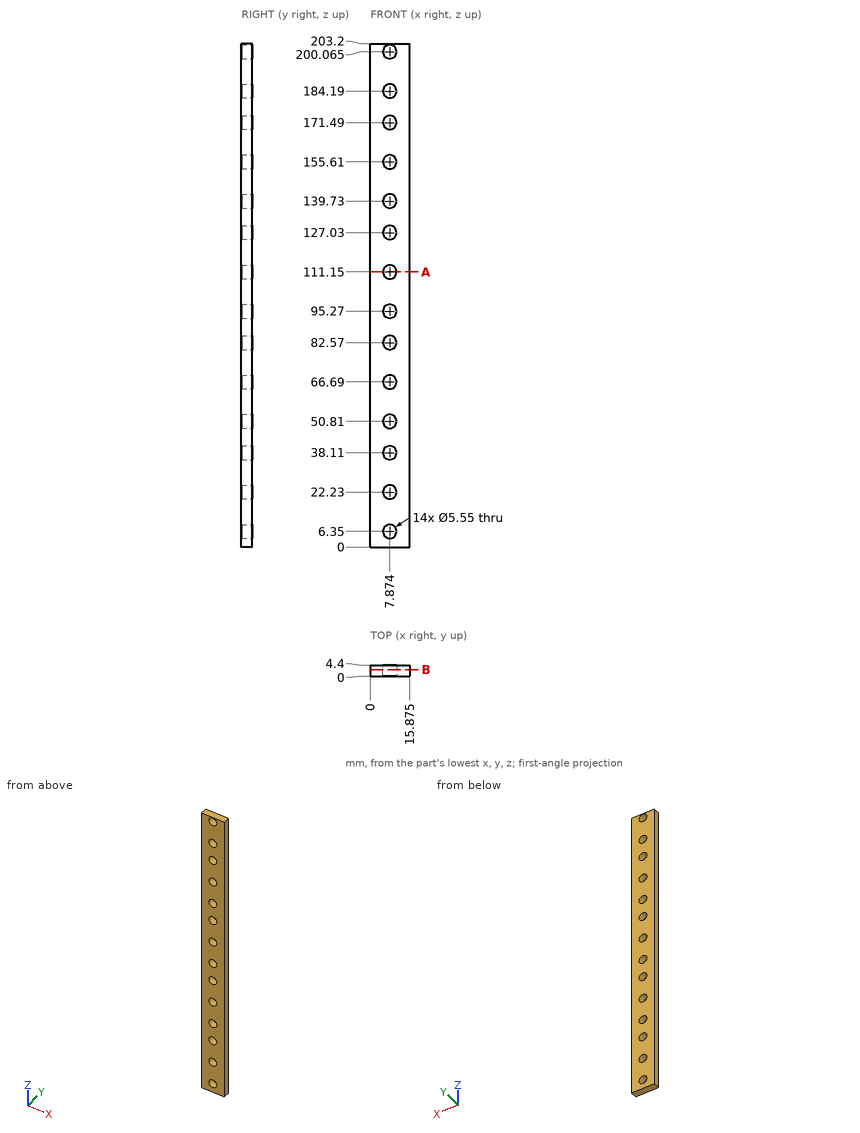
Input: dimensioned drawing with shaded views. Units: mm. Origin: part minimum x, y, z. Give positions to 0.01 mm unless a question says otherwise; leave off trailing zeros. Order: outer loops, then holes, each group sorted by start corner. A loop starts at its lowest first (then second) coordinate and runs counter-clockwise, first axis right, second up. Notation, with made-up numbers: (15.5, -29.75) -> (53.5, -29.75) arc R18 ccw to (53.5, -17.75) -> close; hole circle Ø4 at (-30, 79). An arc over 180 degrees is marked (long way). Use a Markdown table: item, result.
1) Section query B-B, the plane y = 2.55. Count the separate pieces of the cut face and the enclosed holes in it, then the cut area to 3 significant figures.
Answer list:
| item | result |
|---|---|
| separate pieces | 1 |
| enclosed holes | 14 |
| area | 2,890 mm² |
2) Ray query, line 1 along X through (y, z) = (4.05, 21) (3 decimals); line 2 along X through (y, z) = (2.6, 170) (3 decimals). Return the intervals inside material, ascending. Write a range as [from, to].
Answer list:
| item | result |
|---|---|
| line 1 | [0, 5.386], [10.362, 15.875] |
| line 2 | [0, 5.533], [10.215, 15.875] |
3) Section query A-A, the plane z = 111.15. Return the cut outline in (x, y) (3 decimals), then the cut area to 3 significant figures.
Answer list:
| item | result |
|---|---|
| outline | (0, 0) -> (5.099, 0) -> (5.099, 4.4) -> (0, 4.4) -> close; (10.649, 0) -> (15.875, 0) -> (15.875, 4.4) -> (10.649, 4.4) -> close |
| area | 45.4 mm² |
